```python
from build123d import *

# Parameters (mm, degrees)
F0_R        = 4.5
F1_DEPTH    = 25
F2_T1_DEPTH = 25


# Not quite as in the source:
# - a fillet or chamfer that OpenCascade refuses, or shapes differently, is made with other operations: its cross-section is extruded or revolved along the edge and cut away or added


with BuildPart() as f1:
    # F0 (on Front) → F1 (new body)
    with BuildSketch(Plane.XZ):
        with BuildLine():
            ThreePointArc((4.2953224556, -4.1892964806), (5.5575144954, -2.2614227011), (6, 0))
            ThreePointArc((6, 0), (-2.2614227011, 5.5575144954), (-4.2953224556, -4.1892964806))
            ThreePointArc((-4.2953224556, -4.1892964806), (-2.3306888592, -5.5288235133), (0, -6))
            ThreePointArc((0, -6), (2.3306888592, -5.5288235133), (4.2953224556, -4.1892964806))
        make_face()
        Circle(F0_R, mode=Mode.SUBTRACT)
        Polygon((0, -9), (0, -6), (-10, -6), (-20, -6), (-20, -9), align=None)
        with BuildLine():
            ThreePointArc((0, -6), (-2.3306888592, -5.5288235133), (-4.2953224556, -4.1892964806))
            Line((-4.2953224556, -4.1892964806), (-10, -6))
            Line((-10, -6), (0, -6))
        make_face()
    extrude(amount=F1_DEPTH)

    # F2: fillet of radius 5 on 2 edges, made by hand

    # F2_s2 → F2_t1 (join)
    with BuildSketch(Plane.XZ):
        with BuildLine():
            ThreePointArc((-5.9723157586, -0.5757121498), (-6.7770271427, -3.8109383875), (-9.4365815374, -5.8211671413))
            Line((-9.4365815374, -5.8211671413), (-4.2953224556, -4.1892964806))
            ThreePointArc((-4.2953224556, -4.1892964806), (-5.4424807352, -2.5257480964), (-5.9723157586, -0.5757121498))
        make_face()
        with BuildLine():
            ThreePointArc((2.6891271741, -5.3636363636), (0.9099152249, -6.8603913833), (0, -9))
            Line((0, -9), (0, -6))
            ThreePointArc((0, -6), (1.3816985594, -5.8387420812), (2.6891271741, -5.3636363636))
        make_face()
    extrude(amount=F2_T1_DEPTH)


solid = f1.part
```
Work out the finished part from the listing and answer in its coordinate system (mm). A direction names the side the tool comes from. Coordinates: 2 decimals unless noted, no trailing zeros. Loops run counter-clockwise (first coordinate to the right, second up) from the corner with the lowest first, then second, coordinate; pieces in that order, holes last. Notation, with made-up numbers: (61, -9) -> (107, -9) arc R33 cw to (107, 21) -> close; hole circle Ø2 at (20.5, -8.75). An arc over 180 degrees is marked (long way). Answer as CSV lines item,"result".
Q1. The part is cut by section A-A on x = -0.5. Write down the section's boundary in (y, z).
Findings:
outline,"(-25, -9) -> (0, -9) -> (0, -4.47) -> (-25, -4.47) -> close; (-25, 4.47) -> (0, 4.47) -> (0, 5.98) -> (-25, 5.98) -> close"
Q2. The part is cut by section D-D on x = -16.75. Write down the section's boundary in (y, z).
Findings:
outline,"(-25, -9) -> (0, -9) -> (0, -6) -> (-25, -6) -> close"
Q3. Each of these flat-tipped pins is pushed along its axis until it touches: pin 1 (1 mm diameter, centred on x = -9, y = -14.5, fed in from +Z); pin 2 (5 mm diameter, centred on x = -17, y = -8, fed in from +Z); pin 3 (6 mm diameter, centred on x = -3.5, y = -14.5, fed in from +Z). Where does it stop, or does it pass through?
Findings:
pin 1,"stops at z = -5.41"
pin 2,"stops at z = -6"
pin 3,"stops at z = 5.98"
Q4. Find the intervals of material crossed by probe 1 along Z at (x, y) = (-13.75, -11.5); probe 2 along X at (y, z) = (-14, -1.25); probe 3 along X at (y, z) = (-17.5, 2.25), in increasing order.
Findings:
probe 1,"z = -9 to -6"
probe 2,"x = -5.95 to -4.32, 4.32 to 5.87"
probe 3,"x = -5.56 to -3.9, 3.9 to 5.56"
Q5. For a pull along X with two mould halves and no side action, classify faces 3 (the face through (-0.59, -12.32, 4.46)), 4 (the face through (-5, 0, -5)), 5 (the face through (-6.75, -12.32, -3.77)) as +X half, -X half, draft (parallel to the pull), parting line (faces both ways), or undercut.
Findings:
face 3,"undercut"
face 4,"draft"
face 5,"-X half"
Q6. The part is cut by section B-B on z = 2. Write down the section's boundary in (x, y), and give its area (3 significant figures).
Findings:
outline,"(-5.66, -25) -> (-4.03, -25) -> (-4.03, 0) -> (-5.66, 0) -> close; (4.03, -25) -> (5.66, -25) -> (5.66, 0) -> (4.03, 0) -> close"
area,"81.3 mm²"
Q7. The part is cut by section C-C on y = -20.5. Write down the section's boundary in (x, z), and give its area (3 significant figures).
Findings:
outline,"(-20, -9) -> (0, -9) arc R5 cw to (2.69, -5.36) arc R6 ccw (long way) to (-5.97, -0.58) arc R5 cw to (-9.44, -5.82) -> (-10, -6) -> (-20, -6) -> close; hole circle Ø9 at (0, 0)"
area,"124 mm²"
Q8. A tool of negligible diameter and unlimited length cuts with its end or side. For faces 1 (the face through (-15, -12, -6)), 2 (the face through (-5, -25, -5)), from which of +Z, -Z, +X, -X, +Y, -Y can it reach the whole face along a straight path? Write none if from no direction.
Findings:
face 1,"+Z, -X, +Y, -Y"
face 2,"+Z, -Z, +X, -X, -Y"
